```python
from build123d import *

# Parameters (mm, degrees)
F0_R          = 10.795
F0_R_2        = 6.4897
F1_DEPTH      = 20.32
F2_R          = 10.795
F3_DEPTH      = 5.08
F4_W          = 4.6222759372
F4_H          = 14.661224488
F5_DEPTH      = 12.4206
F6_R          = 1.7272
F7_DEPTH      = 10.796
F7_DEPTH_BACK = 25.4
F9_DEPTH      = 4.6222759372
F10_R         = 7.330612244
F11_DEPTH     = 4.6222759372
F12_R         = 2.0828
F13_DEPTH     = 18.7202760372
F14_T4_DEPTH  = 14.661224488
F14_S5_R      = 10.795
F14_T6_DEPTH  = 11
F14_T10_DEPTH = 14.661224488
F14_S11_R     = 10.795
F14_T12_DEPTH = 11
F15_R         = 1.27


# Not quite as in the source:
# - a fillet or chamfer that OpenCascade refuses, or shapes differently, is made with other operations: its cross-section is extruded or revolved along the edge and cut away or added


with BuildPart() as f1:
    # F0 (on Top) → F1 (new body)
    with BuildSketch(Plane.XY):
        Circle(F0_R)
        Circle(F0_R_2, mode=Mode.SUBTRACT)
    extrude(amount=F1_DEPTH)

    # F2 (on face) → F3 (join)
    with BuildSketch(Plane.XY.offset(20.32)):
        Circle(F2_R)
    extrude(amount=F3_DEPTH)

    # F4 (on face) → F5 (join)
    with BuildSketch(Plane.XY.offset(25.4)):
        with Locations((-5.6131379686, 0)):
            Rectangle(F4_W, F4_H)
        with Locations((5.6131379686, 0)):
            Rectangle(F4_W, F4_H)
    extrude(amount=F5_DEPTH)

    # F6 (on Front) → F7 (cut, two sides)
    with BuildSketch(Plane.XZ) as f7_sk:
        with Locations((0, 8.128)):
            Circle(F6_R)
    extrude(amount=F7_DEPTH, mode=Mode.SUBTRACT)
    extrude(f7_sk.sketch, amount=-F7_DEPTH_BACK, mode=Mode.SUBTRACT)

    # F8 (on face) → F9 (join, through all)
    with BuildSketch(Plane(origin=(3.302, 0, 0), x_dir=(0, -1, 0), z_dir=(-1, 0, 0))):
        with BuildLine():
            Line((-7.330612244, 37.8206), (7.330612244, 37.8206))
            ThreePointArc((7.330612244, 37.8206), (0, 45.151212244), (-7.330612244, 37.8206))
        make_face()
    extrude(amount=-F9_DEPTH)

    # F10 (on face) → F11 (join, through all)
    with BuildSketch(Plane(origin=(-7.9242759372, 0, 0), x_dir=(0, -1, 0), z_dir=(-1, 0, 0))):
        with Locations((0, 37.8206)):
            Circle(F10_R)
    extrude(amount=-F11_DEPTH)

    # F12 (on face) → F13 (cut, through all)
    with BuildSketch(Plane(origin=(-7.9242759372, 0, 0), x_dir=(0, -1, 0), z_dir=(-1, 0, 0))):
        with Locations((0, 37.8206)):
            Circle(F12_R)
    extrude(amount=-F13_DEPTH, mode=Mode.SUBTRACT)

    # F14: fillet of radius 7.62 on 2 edges, made by hand


with BuildPart() as f14_tool2:
    # F14_s3 → F14_t4 (new body)
    with BuildSketch(Plane.XZ.offset(7.330612244)):
        with BuildLine():
            ThreePointArc((15.5442759372, 25.4), (10.1561222645, 27.6318463274), (7.9242759372, 33.02))
            Line((7.9242759372, 33.02), (7.9242759372, 25.4))
            Line((7.9242759372, 25.4), (15.5442759372, 25.4))
        make_face()
    extrude(amount=-F14_T4_DEPTH)

    # F14_s5 → F14_t6 (intersect, symmetric)
    with BuildSketch(Plane.XY.offset(29.2)):
        Circle(F14_S5_R)
    extrude(amount=F14_T6_DEPTH, both=True, mode=Mode.INTERSECT)


with BuildPart() as f1_1:
    add(f1.part)

    # F14_t1: union F14_tool2
    add(f14_tool2.part)


with BuildPart() as f14_tool8:
    # F14_s9 → F14_t10 (new body)
    with BuildSketch(Plane.XZ.offset(-7.330612244)):
        with BuildLine():
            ThreePointArc((-15.5442759372, 25.4), (-10.1561222645, 27.6318463274), (-7.9242759372, 33.02))
            Line((-7.9242759372, 33.02), (-7.9242759372, 25.4))
            Line((-7.9242759372, 25.4), (-15.5442759372, 25.4))
        make_face()
    extrude(amount=F14_T10_DEPTH)

    # F14_s11 → F14_t12 (intersect, symmetric)
    with BuildSketch(Plane.XY.offset(29.2)):
        Circle(F14_S11_R)
    extrude(amount=F14_T12_DEPTH, both=True, mode=Mode.INTERSECT)


with BuildPart() as f1_2:
    add(f1_1.part)

    # F14_t7: union F14_tool8
    add(f14_tool8.part)

    # F15
    f15_edges = [f1_2.edges().sort_by_distance(p)[0] for p in [
        (-6.4897, 0, 0),
    ]]
    fillet(f15_edges, radius=F15_R)


solid = f1_2.part
```
Input: part model. Units: mm. Frame: model coordinates. A direction names the side the tool comes from. Round coordinates to 2 decimals unless told otherwise and drop trailing zeros. Order: outer loops, then holes, each group sorted by start corner. A loop starts at its lowest first (then second) coordinate and runs counter-clockwise, first axis right, second up. Notation, with made-up numbers: (-10, -13.75) - (10, -13.75) arc R10 cw to (10, -0.75) - close; hole circle Ø11 at (25, -7). An arc over 180 degrees is marked (long way). One line per question, with ' | ' between items. Start each with the question number.
1) Cut plane D-D, the plane x = -8.5. Return the cut outline in (y, z).
2) Cut plane C-C, the plane z = 12. Return the cut outline in (x, y) (3 decimals), then the cut area to 3 significant figures.
3) Ray query, probe 1 along X at (y, z) = (-2.25, 39); probe 2 along Z at (x, y) = (6.45, 0); probe 3 along Z at (x, y) = (0, -8.1). Return the intervals inside material, ascending.
4) Cut plane B-B, the plane x = 0. Return the cut outline in (y, z) (3 decimals).
5) Contact query for flat-ended pins moving along their axis: P1, Ø5, axis at y = 0, z = 37.82, coming from the -X side; P2, Ø3.5, axis at x = 5, z = 30, coming from the -Y side; P3, Ø2, axis at y = 4, z = 39.5, coming from the +X side; P4, Ø3, axis at x = 0, z = 8.128, coming from the -Y side. Output: stop coordinate, or through.
6) Cut plane A-A, the plane y = 0. Return the cut outline in (x, z) (3 decimals), then the cut area to 3 significant figures.
7) Set-up query: faces 1 (the flat face through (7.924, 2, 39)), 2 (the flat face through (6, -7.331, 32)), 3 (the cylindrical face through (5.995, -2.486, 10.662)). Return all of +Z, -Z, +X, -X, +Y, -Y with unobstructed straight access to the full face (end or side cutting, diameter ignored); none if empty.
8) Pull-direction query (Y, two-part tool) for faces 4 (the cylindrical face through (5.6, 0.5, 35.8)), 5 (the flat face through (0, 0, 25.4)), 6 (the cylindrical face through (-5.65, -0.16, 45.15)); classes: +Y half, -Y half, draft (parallel to the pull), parting line (faces both ways), or undercut.
Worked out:
1) outline: (-6.65, 0) - (6.65, 0) - (6.65, 30.11) - (-6.65, 30.11) - close
2) outline: circle Ø21.59 at (0, 0); hole circle Ø12.979 at (0, 0) | area: 234 mm^2
3) probe 1: x = -7.92 to -3.3, 3.3 to 7.92 | probe 2: z = 20.32 to 35.74, 39.9 to 45.15 | probe 3: z = 0 to 6.4, 9.86 to 25.4
4) outline: (-10.795, 0) - (-7.76, 0) arc R1.27 ccw to (-6.49, 1.27) - (-6.49, 6.401) - (-10.795, 6.401) - close; (-10.795, 9.855) - (-6.49, 9.855) - (-6.49, 20.32) - (6.49, 20.32) - (6.49, 9.855) - (10.795, 9.855) - (10.795, 25.4) - (-10.795, 25.4) - close; (6.49, 1.27) arc R1.27 ccw to (7.76, 0) - (10.795, 0) - (10.795, 6.401) - (6.49, 6.401) - close
5) P1: stops at x = -7.92 | P2: stops at y = -7.33 | P3: stops at x = 7.92 | P4: passes through
6) outline: (-10.795, 0) - (-7.76, 0) arc R1.27 ccw to (-6.49, 1.27) - (-6.49, 20.32) - (6.49, 20.32) - (6.49, 1.27) arc R1.27 ccw to (7.76, 0) - (10.795, 0) - (10.795, 27.061) arc R7.62 cw to (7.924, 33.02) - (7.924, 35.738) - (3.302, 35.738) - (3.302, 25.4) - (-3.302, 25.4) - (-3.302, 35.738) - (-7.924, 35.738) - (-7.924, 33.02) arc R7.62 cw to (-10.795, 27.061) - close; (-7.924, 39.903) - (-3.302, 39.903) - (-3.302, 45.151) - (-7.924, 45.151) - close; (3.302, 39.903) - (7.924, 39.903) - (7.924, 45.151) - (3.302, 45.151) - close | area: 448 mm^2
7) face 1: +Z, +X, +Y, -Y | face 2: +Z, +X, -X, -Y | face 3: -Z
8) face 4: undercut | face 5: draft | face 6: parting line
